Input: dimensioned drawing with shaded views. Units: mm. Origin: part minimum x, y, z. A direction names the side the tool comes from. Round coordinates to 2 decimals unless told otherwise and drop trailing zeros. Loops run counter-clockwise (first coordinate to the right, second up) from the corner with the lowest first, then second, coordinate; pieces in that order, holes last. Notation, with made-up numbers: M -19,-5.75 L -13,-5.75 A9 cw -13,0.25 Z; hole C 72,10 d4. An arc over 180 degrees is marked long. Put each result on its own line as item: value. Start each with the question number.
1) Section B-B on y = 22.25. Output: boundary loops of the cut face in (x, z), plus the area to 3 significant figures.
2) Pin query (flat end, axial travel): pin 1 (1 mm diameter, centred on y = 15, z = 1.5, fed in from -X); pin 2 (0.7 mm diameter, centred on x = 0.5, y = 14.5, fed in from -Z); pin 3 (0.7 mm diameter, centred on x = 1, y = 2.5, fed in from +Z); pin 4 (1.2 mm diameter, centred on x = 1, y = 3, fed in from -Z). Return the tip coordinate at first contact, or that it passes through.
3) Reachability of the marked faces 3, 4 and 5 from +Z, -Z, +X, -X, +Y, -Y: full face, straight path, thin tool, end or side. Return the list, or none.
4) Draft query along Z for the marked faces 1 and 2. Return one class per face: +Z half, -Z half, draft (parallel to the pull), parting line (faces both ways), or undercut.
5) Line query: probe 1 along Y at (x, z) = (0.8, 5); probe 2 along X at (y, z) = (25, 7.5); probe 3 along Z at (x, y) = (1.8, 23.5). Output: solid intervals per line, ascending.
6) Section C-C on y = 14.75. Output: boundary loops of the cut face in (x, z).
7) Section A-A on z = 5. Output: boundary loops of the cut face in (x, y).
8) Section D-D on z = 8.25. Output: boundary loops of the cut face in (x, y), plus the area to 3 significant figures.
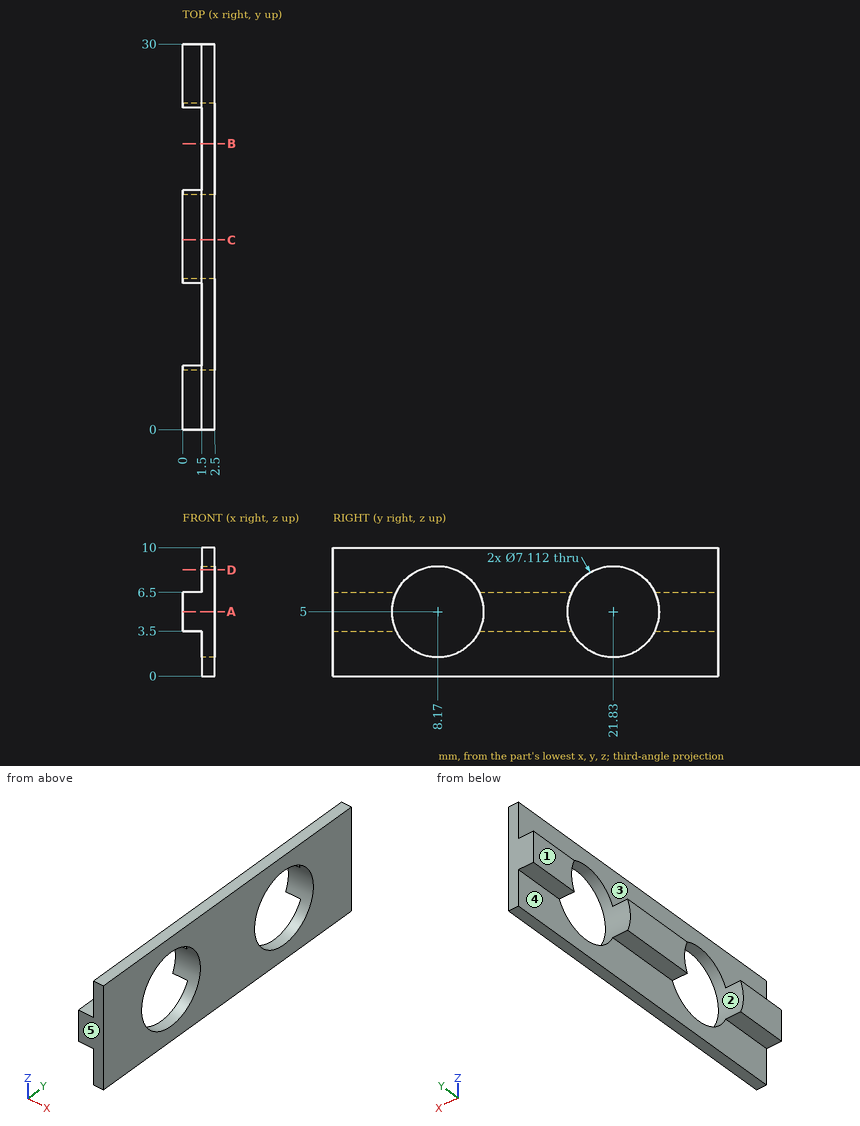
Geometry results:
1. outline: M 1.5,0 L 2.5,0 L 2.5,1.47 L 1.5,1.47 Z; M 1.5,8.53 L 2.5,8.53 L 2.5,10 L 1.5,10 Z
1. area: 2.94 mm²
2. pin 1: stops at x = 1.5
2. pin 2: stops at z = 3.5
2. pin 3: stops at z = 6.5
2. pin 4: stops at z = 0
3. face 3: +Z, -X, +Y, -Y
3. face 4: -Z, -X, +Y, -Y
3. face 5: +Z, -Z, +X, -X, -Y
4. face 1: draft
4. face 2: undercut
5. probe 1: y = 0 to 4.61, 11.73 to 18.27, 25.39 to 30
5. probe 2: x = 1.5 to 2.5
5. probe 3: z = 0 to 1.86, 8.14 to 10
6. outline: M 0,3.5 L 1.5,3.5 L 1.5,0 L 2.5,0 L 2.5,10 L 1.5,10 L 1.5,6.5 L 0,6.5 Z
7. outline: M 0,0 L 2.5,0 L 2.5,4.61 L 0,4.61 Z; M 0,11.73 L 2.5,11.73 L 2.5,18.27 L 0,18.27 Z; M 0,25.39 L 2.5,25.39 L 2.5,30 L 0,30 Z
8. outline: M 1.5,0 L 2.5,0 L 2.5,6.73 L 1.5,6.73 Z; M 1.5,9.61 L 2.5,9.61 L 2.5,20.39 L 1.5,20.39 Z; M 1.5,23.27 L 2.5,23.27 L 2.5,30 L 1.5,30 Z
8. area: 24.2 mm²
